```python
from build123d import *

# Parameters (mm, degrees)
SKETCH1_R                = 8.022684963
SKETCH1_R_2              = 4.06906829
BOSS_EXTRUDE1_DEPTH      = 9
CUT_EXTRUDE2_DEPTH       = 80
CUT_EXTRUDE2_DEPTH_BACK  = 80
CUT_EXTRUDE15_DEPTH      = 68.428154516
CUT_EXTRUDE15_DEPTH_BACK = 68.428154516


with BuildPart() as part:
    # Sketch1 → Boss-Extrude1 (new body)
    with BuildSketch(Plane(origin=(0, 0, 0), x_dir=(1, 0, 0), z_dir=(0, 1, 0))):
        with BuildLine():
            Line((-2.221076805, 65.28335408), (-1.171915361, 65.28335408))
            ThreePointArc((-1.171915361, 65.28335408), (6.823214902, 61.838345283), (9.810473513, 53.661152641))
            Line((9.810473513, 53.661152641), (7.206522245, 7.699180155))
            ThreePointArc((7.206522245, 7.699180155), (4.713869394, 2.337050101), (-0.780669663, 0.151690292))
            Line((-0.780669663, 0.151690292), (-2.221076805, 0.151690292))
            Line((-2.221076805, 0.151690292), (-3.661483948, 0.151690292))
            ThreePointArc((-3.661483948, 0.151690292), (-9.156023005, 2.337050101), (-11.648675856, 7.699180155))
            Line((-11.648675856, 7.699180155), (-14.252627123, 53.661152641))
            ThreePointArc((-14.252627123, 53.661152641), (-11.265368512, 61.838345283), (-3.27023825, 65.28335408))
            Line((-3.27023825, 65.28335408), (-2.221076805, 65.28335408))
        make_face()
        with Locations(Location((-2.221076805, 52.32335408, 0), (0, 0, 270))):
            Circle(SKETCH1_R, mode=Mode.SUBTRACT)
        with Locations(Location((-2.221076805, 10.201686469, 0), (0, 0, 270))):
            Circle(SKETCH1_R_2, mode=Mode.SUBTRACT)
    extrude(amount=BOSS_EXTRUDE1_DEPTH)

    # Sketch2 → Cut-Extrude2 (cut, two sides: drawn at the far end of the back side and taken through both)
    with BuildSketch(Plane(origin=(0, 0, 0), x_dir=(0, 0, -1), z_dir=(1, 0, 0)).offset(-CUT_EXTRUDE2_DEPTH_BACK)):
        with BuildLine():
            add(Edge.make_bspline(
                [(15.233518693, 4.5), (20.997577491, 4.003468068), (26.535168731, 1.567737081), (32.11164194, 0)],
                knots=[0.310739068, 0.310739068, 0.310739068, 0.310739068, 1, 1, 1, 1], degree=3))
            Line((32.11164194, 0), (0.151690292, 0))
            Line((0.151690292, 0), (0.151690292, 4.5))
            Line((0.151690292, 4.5), (7.699180155, 4.5))
            Line((7.699180155, 4.5), (15.233518693, 4.5))
        make_face()
    extrude(amount=CUT_EXTRUDE2_DEPTH + CUT_EXTRUDE2_DEPTH_BACK, mode=Mode.SUBTRACT)

    # Sketch3 → Cut-Extrude15 (cut, two sides: drawn at the far end of the back side and taken through both)
    with BuildSketch(Plane(origin=(0, 0, 0), x_dir=(0, 0, -1), z_dir=(1, 0, 0)).offset(-CUT_EXTRUDE15_DEPTH_BACK)):
        with BuildLine():
            Line((65.441158073, 9.059719613), (65.441158073, 9.358577967))
            Line((65.441158073, 9.358577967), (15.059583295, 9.985835555))
            Line((15.059583295, 9.985835555), (14.793593064, 9.985835555))
            Line((14.793593064, 9.985835555), (0, 9.985835555))
            Line((0, 9.985835555), (0, 8.994860535))
            Line((0, 8.994860535), (15.059583295, 8.994860535))
            add(Edge.make_bspline(
                [(15.059583295, 8.994860535), (20.823642093, 8.498328604), (26.361233333, 6.062597616), (31.937706542, 4.494860535)],
                knots=[0.310739068, 0.310739068, 0.310739068, 0.310739068, 1, 1, 1, 1], degree=3))
            Line((31.937706542, 4.494860535), (65.441158073, 4.533727355))
            Line((65.441158073, 4.533727355), (65.441158073, 9.059719613))
        make_face()
    extrude(amount=CUT_EXTRUDE15_DEPTH + CUT_EXTRUDE15_DEPTH_BACK, mode=Mode.SUBTRACT)


solid = part.part
```
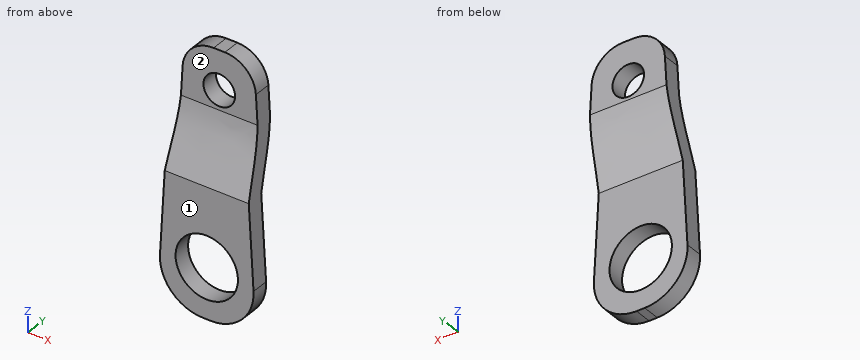
Check sheet for the modelled part. Datum: model origin and axes. Units: mm. Face numbers are marked on the shaded views. A direction names the side the tool comes from. Coordinates: 2 decimals unless noted, no trailing zeros. Write each loop counter-clockwise with the first axis right and the second up, starting at its lowest first coordinate (ties: lowest second). Pieces come first, ordered by that corner, then holes. Notation, with made-up numbers: (27, 39.25) -> (77, 39.25) arc R29 cw to (77, 60.25) -> close; hole circle Ø10 at (87, 36.25). An arc over 180 degrees is marked (long way). Use a Markdown table: item, result.
1. Sectioned sample at A-A (z = -52). Enter the section's corners in (x, y).
Reported:
| item | result |
|---|---|
| outline | (-14.16, 0) -> (-10.24, 0) -> (-10.24, 4.52) -> (-14.16, 4.52) -> close; (5.8, 0) -> (9.72, 0) -> (9.72, 4.52) -> (5.8, 4.52) -> close |
2. Tool access check on the marked faces 1 and 2. Record the directions out of +Z, -Z, +X, -X, +Y, -Y that give a thin tool (end or side, any length) a straight path to the whole face; none if there is none.
Reported:
| item | result |
|---|---|
| face 1 | +Z, -Z, +X, -X, -Y |
| face 2 | +Z, +X, -X, -Y |
3. Go/stop test with flat-tipped pins: pin 1 Ø5 at (x, z) = (-7, -55.5) entering from +Y; pin 2 Ø3 at (x, y) = (-10, 4) entering from -Z; pin 3 Ø3 at (y, z) = (7.5, -33) entering from +X; pin 4 Ø12 at (x, z) = (-10, -36.5) entering from +Y. Record where each tip stops, or that it passes through.
Reported:
| item | result |
|---|---|
| pin 1 | stops at y = 4.52 |
| pin 2 | stops at z = -63.96 |
| pin 3 | passes through |
| pin 4 | stops at y = 4.92 |
4. Sectioned sample at D-D (z = -33). Enter the section's corners in (x, y), plus the area to 3 significant figures.
Reported:
| item | result |
|---|---|
| outline | (-13.08, 0) -> (8.64, 0) -> (8.64, 4.5) -> (-13.08, 4.5) -> close |
| area | 97.7 mm2 |
5. Sectioned sample at B-B (x = 1.25). Give the number of separate pieces and of enclosed holes in the cut face, plus the area to 3 significant figures.
Reported:
| item | result |
|---|---|
| separate pieces | 3 |
| enclosed holes | 0 |
| area | 206 mm2 |
6. Scan lines: line 1 along Y through (x, z) = (-8.25, -36); line 2 along X through (y, z) = (2, -48); line 3 along X through (y, z) = (8.5, -9). Record each from-to range of solid material in increasing order.
Reported:
| item | result |
|---|---|
| line 1 | y = 0 to 4.5 |
| line 2 | x = -13.93 to -8.98, 4.54 to 9.49 |
| line 3 | x = -11.72 to -6.11, 1.67 to 7.28 |
7. Sectioned sample at C-C (z = -13). Enter the section's corners in (x, y).
Reported:
| item | result |
|---|---|
| outline | (-11.95, 4.5) -> (-5.18, 4.5) -> (-5.18, 8.99) -> (-11.95, 8.99) -> close; (0.73, 4.5) -> (7.51, 4.5) -> (7.51, 8.99) -> (0.73, 8.99) -> close |
